Answer from the drawing. Dimensions are ordinates in mm from the lowest x, y and z of the part. A direction names the side the tool comes from. Coordinates: 2 decimals unless noted, no trailing zeros. Write each loop counter-clockwise with the first axis right and the second up, starting at its lowest first coordinate (ties: lowest second). Pieces come first, ordered by that corner, then holes. Notation, with made-up numbers: (0.5, 32) - (13.5, 32) arc R19 ccw to (13.5, 47) - close; hole circle Ø2 at (78, 33.25). An arc over 180 degrees is marked (long way). Use a Markdown table: item, result.
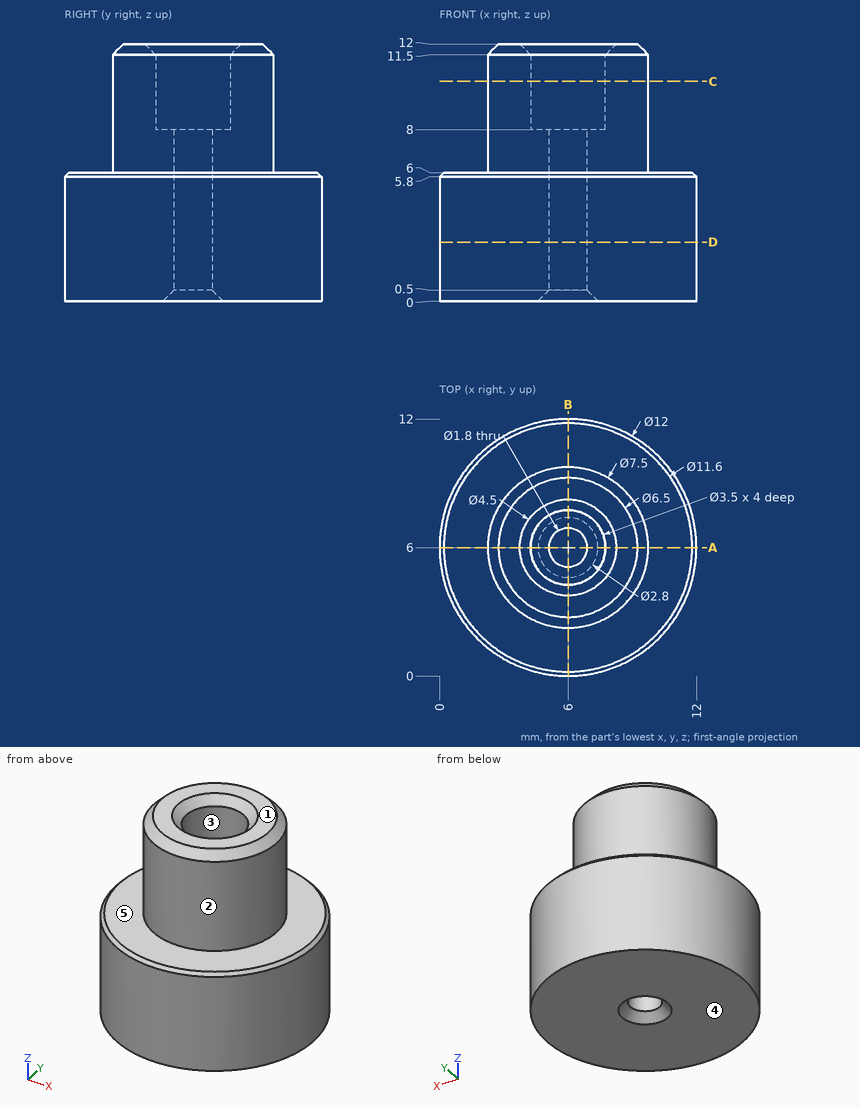
(1) For the marked faces 4 and 5, determine the directions among +Z, -Z, +X, -X, +Y, -Y from which every point of the face is accessible in a straight line to the end or side of a thin tool.
Report:
| item | result |
|---|---|
| face 4 | -Z, +X, -X, +Y, -Y |
| face 5 | +Z |
(2) A cutting plane is placed at C-C, the plane z = 10.25. Write down the section's boundary in (x, y).
Report:
| item | result |
|---|---|
| outline | circle Ø7.5 at (6, 6); hole circle Ø3.5 at (6, 6) |
(3) Each of these flat-tipped pins is pushed along its axis until it touches: P1, Ø1, axis at x = 5.5, y = 6, coming from the +Z side; P2, Ø2, axis at x = 6, y = 6, coming from the -Z side; P3, Ø5, axis at x = 2.5, z = 7, coming from the -Y side. Where does it stop, or does it pass through?
Report:
| item | result |
|---|---|
| P1 | stops at z = 8 |
| P2 | stops at z = 0.4 |
| P3 | stops at y = 0.14 |
(4) A cutting plane is placed at A-A, the plane y = 6. Write down the section's boundary in (x, z), and give its area (3 significant figures).
Report:
| item | result |
|---|---|
| outline | (0, 0) - (4.6, 0) - (5.1, 0.5) - (5.1, 8) - (4.25, 8) - (4.25, 11.5) - (3.75, 12) - (2.75, 12) - (2.25, 11.5) - (2.25, 6) - (0.2, 6) - (0, 5.8) - close; (6.9, 0.5) - (7.4, 0) - (12, 0) - (12, 5.8) - (11.8, 6) - (9.75, 6) - (9.75, 11.5) - (9.25, 12) - (8.25, 12) - (7.75, 11.5) - (7.75, 8) - (6.9, 8) - close |
| area | 87.8 mm² |
(5) Straight lines are drawn through the part: L1, parallel to Y at x = 6, z = 2.5; L2, parallel to Y at x = 6, z = 8.75; L3, parallel to Z at x = 2, y = 4. For each, find the intervals that lie inside material, in ascending order.
Report:
| item | result |
|---|---|
| L1 | y = 0 to 5.1, 6.9 to 12 |
| L2 | y = 2.25 to 4.25, 7.75 to 9.75 |
| L3 | z = 0 to 6 |
(6) A cutting plane is placed at D-D, the plane z = 2.75. Write down the section's boundary in (x, y).
Report:
| item | result |
|---|---|
| outline | circle Ø12 at (6, 6); hole circle Ø1.8 at (6, 6) |
(7) The mould has two halves that part along X. Classify the marked faces 1, 2 and 3: pulls with the +X half, pulls with the -X half, needs draft (parallel to the pull), parting line crosses it, or undercut.
Report:
| item | result |
|---|---|
| face 1 | needs draft |
| face 2 | parting line crosses it |
| face 3 | undercut |
